from build123d import *

# Parameters (mm, degrees)
F0_R     = 2.2225
F0_R_2   = 1.905
F0_R_3   = 8.73125
F1_DEPTH = 5.08
F2_R     = 3.175
F3_T     = -2.032
F4_R     = 4.92125
F4_R_2   = 1.905
F4_R_3   = 2.2225
F5_DEPTH = 6.35


with BuildPart() as f1:
    # F0 (on Top) → F1 (new body)
    with BuildSketch(Plane.XY):
        with BuildLine():
            ThreePointArc((39.6875, 60.325), (38.7575640303, 62.5700640303), (36.5125, 63.5))
            Line((36.5125, 63.5), (-36.5125, 63.5))
            ThreePointArc((-36.5125, 63.5), (-38.7575640303, 62.5700640303), (-39.6875, 60.325))
            Line((-39.6875, 60.325), (-39.6875, -60.325))
            ThreePointArc((-39.6875, -60.325), (-38.7575640303, -62.5700640303), (-36.5125, -63.5))
            Line((-36.5125, -63.5), (36.5125, -63.5))
            ThreePointArc((36.5125, -63.5), (38.7575640303, -62.5700640303), (39.6875, -60.325))
            Line((39.6875, -60.325), (39.6875, 60.325))
        make_face()
        with Locations((0, -40.64)):
            Circle(F0_R, mode=Mode.SUBTRACT)
        with Locations((-17.145, 0)):
            Circle(F0_R_2, mode=Mode.SUBTRACT)
        Circle(F0_R_3, mode=Mode.SUBTRACT)
        with Locations((17.145, 0)):
            Circle(F0_R_2, mode=Mode.SUBTRACT)
        with Locations((0, 40.64)):
            Circle(F0_R, mode=Mode.SUBTRACT)
    extrude(amount=-F1_DEPTH)

    # F2
    f2_edges = [f1.edges().sort_by_distance(p)[0] for p in [
        (0, -63.5, 0),
    ]]
    fillet(f2_edges, radius=F2_R)

    # F3
    f3_openings = [f1.faces().sort_by_distance(p)[0] for p in [
        (38.189855, 0, -5.08),
    ]]
    offset(amount=F3_T, openings=f3_openings)

    # F4 (on face) → F5 (join)
    with BuildSketch(Plane.XY):
        with Locations((-17.145, 0)):
            Circle(F4_R)
        with Locations((-17.145, 0)):
            Circle(F4_R_2, mode=Mode.SUBTRACT)
        with Locations((17.145, 0)):
            Circle(F4_R)
        with Locations((17.145, 0)):
            Circle(F4_R_2, mode=Mode.SUBTRACT)
        with Locations((0, 40.64)):
            Circle(F4_R)
        with Locations((0, 40.64)):
            Circle(F4_R_3, mode=Mode.SUBTRACT)
        with Locations((0, -40.64)):
            Circle(F4_R)
        with Locations((0, -40.64)):
            Circle(F4_R_3, mode=Mode.SUBTRACT)
    extrude(amount=-F5_DEPTH)


solid = f1.part
Build history of the part. All positions in model axes, mm. A direction names the side the tool comes from. Round coordinates to 2 decimals unless told otherwise and drop trailing zeros. Loops run counter-clockwise (first coordinate to the right, second up) from the corner with the lowest first, then second, coordinate; pieces in that order, holes last. Notation, with made-up numbers: (83.5, 66.5) -> (108.5, 66.5) arc R17 cw to (108.5, 94.5) -> close; hole circle Ø10 at (84.5, 86.25). An arc over 180 degrees is marked (long way). One line per item, written item: value. Start each with the question number.
Q1. Cut at D-D on y = 0. Count the separate pieces of the cut face and the enclosed holes in it, plus the area to 3 significant figures.
Q2. Cut at B-B on x = 32.5. List the corners of the cut face in (y, z) (3 decimals).
Q3. Drop flat-ended pins along their axis: pin 1 Ø3 at (y, z) = (42, -1.5) entering from -X; pin 2 Ø6 at (x, y) = (-17.5, 21.5) entering from -Z. Give the stop position or say it passes through.
Q4. 3-axis set-ups, long thin cutter, end or side, ignore diameter. For faces 4 (the face through (2, 42, -6.35)), 5 (the face through (-22.06, 0.22, -4.16)): which of +Z, -Z, +X, -X, +Y, -Y reach the whole face in a straight line?
Q5. Probe line 1 along X through (y, z) = (19.5, -4); line 2 along X through (y, z) = (44.5, -5); line 3 along Y through (x, z) = (-13, -2.25). List the from-to ranges inside material, lowest first.
Q6. Two-plate mould, pull along X, no slides. Class faces 1 (the face through (-6.93, -5.31, -2.5)), 2 (the face through (38.78, 0.84, -0.95)), 3 (the face through (38, 0, -5.08)): released by +X, released by -X, zero draft, split by the parting line, or undercut.
Computed:
1. separate pieces: 4
1. enclosed holes: 0
1. area: 183 mm²
2. outline: (-63.5, -5.08) -> (-61.468, -5.08) -> (-61.468, -3.175) arc R1.143 cw to (-60.325, -2.032) -> (60.325, -2.032) arc R1.143 cw to (61.468, -3.175) -> (61.468, -5.08) -> (63.5, -5.08) -> (63.5, -3.175) arc R3.175 ccw to (60.325, 0) -> (-60.325, 0) arc R3.175 ccw to (-63.5, -3.175) -> close
3. pin 1: x = -39.68
3. pin 2: z = -2.03
4. face 4: -Z, +X, -X, +Y, -Y
4. face 5: -Z
5. line 1: -39.69 to -37.66, 37.66 to 39.69
5. line 2: -39.69 to -37.66, -3.05 to 3.05, 37.66 to 39.69
5. line 3: -63.36 to -61, -2.65 to 2.65, 61 to 63.36
6. face 1: undercut
6. face 2: released by +X
6. face 3: zero draft
